```python
from build123d import *

# Parameters (mm, degrees)
F1_DEPTH = 10
F3_D     = 5.5
F5_D     = 4.2
F5_DEPTH = 14.4
F5_TIP   = 1.2618073


with BuildPart() as f1:
    # F0 (on Front) → F1 (new body)
    with BuildSketch(Plane.XZ):
        Polygon((-40, 26), (-40, -26), (40, -26), (40, 26), (20, 26), (20, 6), (-20, 6), (-20, 26), align=None)
    extrude(amount=F1_DEPTH)

    # F3 (through all)
    with Locations(Plane.XZ.offset(10)):
        with Locations((-30, 16), (-10, -4), (10, -4), (30, 16)):
            Hole(F3_D / 2)

    # F5
    with Locations(Plane.XY.offset(6)):
        with Locations((0, -5.0000003539)):
            Hole(F5_D / 2, depth=F5_DEPTH)
            with Locations((0, 0, -(F5_DEPTH + F5_TIP / 2))):  # 118° drill point
                Cone(0, F5_D / 2, F5_TIP, mode=Mode.SUBTRACT)


solid = f1.part
```
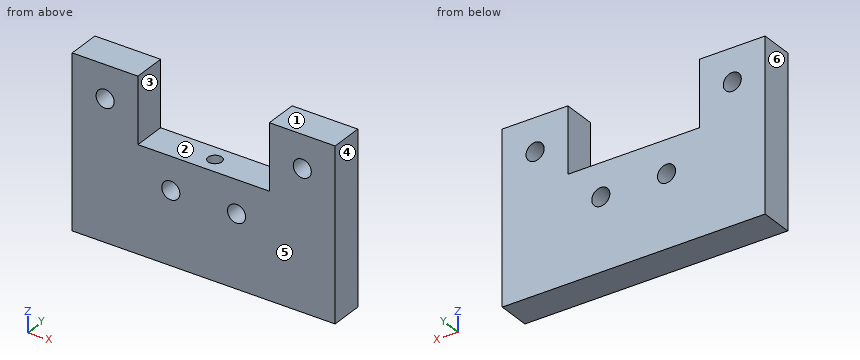
Can you work these out from the model? Positions are in its coordinate system, mm. Face numbers are marked on the shaded views. A direction names the side the tool comes from. Coordinates: 2 decimals unless noted, no trailing zeros. Write each loop counter-clockwise with the first axis right and the second up, starting at its lowest first coordinate (ties: lowest second). Pieces come first, ordered by that corner, then holes. Notation, with made-up numbers: M -12,70.25 L 26,70.25 A34 ccw 26,101.25 Z; hole C 56,68.25 d5. An arc over 180 degrees is marked long. Write item = value, one per line. Start each with the question number.
Q1. I'm going to push flat-ended pins straight in: pin 1 (5 mm diameter, centred on x = 30, z = 16, fed in from -Y); pin 2 (5.5 mm diameter, centred on x = 0, y = -5, fed in from +Z). Where does each tip first touch, or does it pass through?
Q2. If we section it at C-C, the plane x = -10: Write out the boundary of the cut face in (y, z).
Q3. If I drill on L1, parallel to Y at x = 0, z = 1; L2, parallel to X at y = -8.25, z = -3.5; L3, parallel to Z at x = 10, y = -7.5, over which ranges is the centre line in solid material (lowest first)? Write a range as [from, to].
Q4. If we section it at D-D, the plane z = 16: Write out the boundary of the cut face in (x, y), then the cut area to 3 significant figures.
Q5. On a 3-axis mill with a long thin cutter (end or side, diameter ignored), from which of +Z, -Z, +X, -X, +Y, -Y can I reach the whole of each face in a straight line? I mean the marked faces 1 and 2. Say none if no direction works.
Q6. Thinking about a two-plate mould opening in X: for the marked faces 3, 4, 5 and 6, which applies, released by +X, released by -X, zero draft, split by the parting line, or undercut?
Q7. If we section it at A-A, the plane z = -4: Write out the boundary of the cut face in (x, y).
Q8. If we section it at B-B, the plane z = 22.5: Write out the boundary of the cut face in (x, y).
Check sheet entries:
q1.pin_1 = through
q1.pin_2 = 6
q2.outline = M -10,-26 L 0,-26 L 0,-6.75 L -10,-6.75 Z; M -10,-1.25 L 0,-1.25 L 0,6 L -10,6 Z
q3.L1 = [-10, -7.1], [-2.9, 0]
q3.L2 = [-40, -12.7], [-7.3, 7.3], [12.7, 40]
q3.L3 = [-26, -6.75], [-1.25, 6]
q4.outline = M -40,-10 L -32.75,-10 L -32.75,0 L -40,0 Z; M -27.25,-10 L -20,-10 L -20,0 L -27.25,0 Z; M 20,-10 L 27.25,-10 L 27.25,0 L 20,0 Z; M 32.75,-10 L 40,-10 L 40,0 L 32.75,0 Z
q4.area = 290 mm²
q5.face_1 = +Z, +X, -X, +Y, -Y
q5.face_2 = +Z, +Y, -Y
q6.face_3 = undercut
q6.face_4 = released by +X
q6.face_5 = zero draft
q6.face_6 = released by -X
q7.outline = M -40,-10 L -12.75,-10 L -12.75,0 L -40,0 Z; M -7.25,-10 L 7.25,-10 L 7.25,0 L -7.25,0 Z; M 12.75,-10 L 40,-10 L 40,0 L 12.75,0 Z; hole C 0,-5 d4.2
q8.outline = M -40,-10 L -20,-10 L -20,0 L -40,0 Z; M 20,-10 L 40,-10 L 40,0 L 20,0 Z
